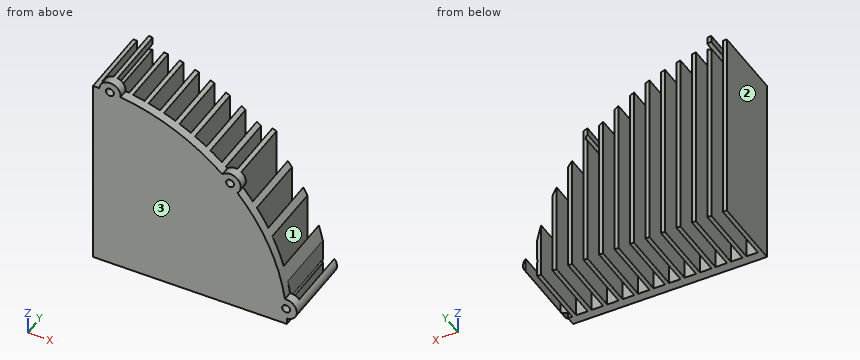
from build123d import *

# Parameters (mm, degrees)
BOSS_EXTRUDE1_DEPTH = 1000
SKETCH2_R           = 3
CUT_EXTRUDE2_DEPTH  = 1016.012315196


with BuildPart() as part:
    # Sketch1 → Boss-Extrude1 (new body)
    with BuildSketch(Plane.XY):
        Polygon((11.571428571, 55), (11.571428571, 7), (3, 7), (3, 55), (0, 55), (0, 7), (0, 0), (165, 0), (165, 7), (165, 10), (165, 55), (162, 55), (162, 7), (153.428571429, 7), (153.428571429, 55), (150.428571429, 55), (150.428571429, 7), (141.857142857, 7), (141.857142857, 55), (138.857142857, 55), (138.857142857, 7), (130.285714286, 7), (130.285714286, 55), (127.285714286, 55), (127.285714286, 7), (118.714285714, 7), (118.714285714, 55), (115.714285714, 55), (115.714285714, 7), (107.142857143, 7), (107.142857143, 55), (104.142857143, 55), (104.142857143, 7), (95.571428571, 7), (95.571428571, 55), (92.571428571, 55), (92.571428571, 7), (84, 7), (84, 55), (81, 55), (81, 7), (72.428571429, 7), (72.428571429, 55), (69.428571429, 55), (69.428571429, 7), (60.857142857, 7), (60.857142857, 55), (57.857142857, 55), (57.857142857, 7), (49.285714286, 7), (49.285714286, 55), (46.285714286, 55), (46.285714286, 7), (37.714285714, 7), (37.714285714, 55), (34.714285714, 55), (34.714285714, 7), (26.142857143, 7), (26.142857143, 55), (23.142857143, 55), (23.142857143, 7), (14.571428571, 7), (14.571428571, 55), align=None)
    extrude(amount=BOSS_EXTRUDE1_DEPTH)

    # Sketch2 → Cut-Extrude2 (cut, through all)
    with BuildSketch(Plane.XZ):
        with BuildLine():
            Line((0, 1000), (0, 145))
            ThreePointArc((0, 145), (2.326211237, 144.981339286), (4.651823732, 144.925361949))
            ThreePointArc((4.651823732, 144.925361949), (13.33482864, 152.417788808), (20.584872923, 143.531400769))
            ThreePointArc((20.584872923, 143.531400769), (61.279647952, 131.41462912), (96.71973071, 108.02913353))
            ThreePointArc((96.71973071, 108.02913353), (108.187337522, 108.187337522), (108.02913353, 96.71973071))
            ThreePointArc((108.02913353, 96.71973071), (131.41462912, 61.279647952), (143.531400769, 20.584872923))
            ThreePointArc((143.531400769, 20.584872923), (152.417788808, 13.33482864), (144.925361949, 4.651823732))
            ThreePointArc((144.925361949, 4.651823732), (144.981339286, 2.326211237), (145, 0))
            Line((145, 0), (165, 0))
            Line((165, 0), (165, 1000))
            Line((165, 1000), (0, 1000))
        make_face()
        with BuildLine():
            ThreePointArc((144.678768073, 9.646453687), (146.649550209, 10.599398525), (147.448231223, 12.637582698))
            ThreePointArc((147.448231223, 12.637582698), (146.46353407, 14.859868557), (144.155861599, 15.623302043))
            ThreePointArc((144.155861599, 15.623302043), (144.448231223, 12.637582698), (144.678768073, 9.646453687))
        make_face()
        with BuildLine():
            ThreePointArc((144.678768073, 9.646453687), (144.448231223, 12.637582698), (144.155861599, 15.623302043))
            ThreePointArc((144.155861599, 15.623302043), (141.459647129, 12.37611547), (144.678768073, 9.646453687))
        make_face()
        with BuildLine():
            ThreePointArc((104.629745412, 100.387331745), (105.296146522, 101.368112079), (105.530483272, 102.530483272))
            ThreePointArc((105.530483272, 102.530483272), (103.664181958, 105.308023063), (100.387331745, 104.629745412))
            ThreePointArc((100.387331745, 104.629745412), (102.530483272, 102.530483272), (104.629745412, 100.387331745))
        make_face()
        with BuildLine():
            ThreePointArc((104.629745412, 100.387331745), (102.530483272, 102.530483272), (100.387331745, 104.629745412))
            ThreePointArc((100.387331745, 104.629745412), (100.409162928, 100.409162928), (104.629745412, 100.387331745))
        make_face()
        with Locations(Location((12.637582698, 144.448231223, 0), (0, 0, 270))):
            Circle(SKETCH2_R)
    extrude(amount=-CUT_EXTRUDE2_DEPTH, mode=Mode.SUBTRACT)


solid = part.part
Read the model definition and answer for the solid it produces. Units are mm, in the model's axes. Face numbers are marked on the shaded views. Round coordinates to 2 decimals unless told otherwise and drop trailing zeros. Order: outer loops, then holes, each group sorted by start corner. A loop starts at its lowest first (then second) coordinate and runs counter-clockwise, first axis right, second up. Notation, with made-up numbers: (-34, 59) - (-27, 59) arc R35 ccw to (-27, 91) - close; hole circle Ø9 at (48, -9). An arc over 180 degrees is marked (long way). Use one line per item in the form item = value. Start each with the question number.
(1) Determine the mould class of the marked faces 1, 2 and 3 for opening direction X: +X half, -X half, draft (parallel to the pull), parting line (faces both ways), or undercut.
(2) The part is cut by section D-D (x = 78.5). Give the vertices of the cut face in (y, z), then the cut area to 3 significant figures.
(3) The part is cut by section A-A (y = 47). Count the separate pieces of the cut face and the enclosed holes in it, then the cut area to 3 significant figures.
(4) Find the intervals of material crossed by line 1 along X through (y, z) = (32.5, 135.5); line 2 along X through (y, z) = (27, 144); line 3 along Y through (x, z) = (101, 108), in increasing order. Write a range as from..to.
(5) Flat-ended cylindrical pins translate along their axes: pin 1 Ø5 at (y, z) = (30, 131.5) entering from +X; pin 2 Ø4.5 at (x, z) = (136.5, 17.5) entering from +Y; pin 3 Ø6 at (x, y) = (55.5, 15.5) entering from +Z; pin 4 Ø5 at (x, y) = (89.5, 25.5) entering from -Z. Find the tip coordinate at first contact, or state that the pin passes through.
(6) The part is cut by section C-C (x = 52). Give the vertices of the cut face in (y, z), then the cut area to 3 significant figures.
Checked values:
q1.face_1 = undercut
q1.face_2 = -X half
q1.face_3 = draft
q2.outline = (0, 0) - (7, 0) - (7, 121.91) - (0, 121.91) - close
q2.area = 853 mm^2
q3.separate_pieces = 15
q3.enclosed_holes = 0
q3.area = 4,500 mm^2
q4.line_1 = 0..3, 11.57..14.57, 23.14..26.14, 34.71..37.71, 46.29..49.29
q4.line_2 = 0..3
q4.line_3 = 0..7
q5.pin_1 = 60.86
q5.pin_2 = 7
q5.pin_3 = 132.96
q5.pin_4 = through
q6.outline = (0, 0) - (7, 0) - (7, 135.36) - (0, 135.36) - close
q6.area = 947 mm^2
